Drawing for the job (mm, zero at the part's lowest x, y, z). Give positions to 0.01 mm unless a question says otherwise; leave off trailing zeros. Write each loop counter-clockwise with the first axis right and the second up, starting at its lowest first coordinate (ties: lowest second). Pieces come first, ordered by that corner, then holes.
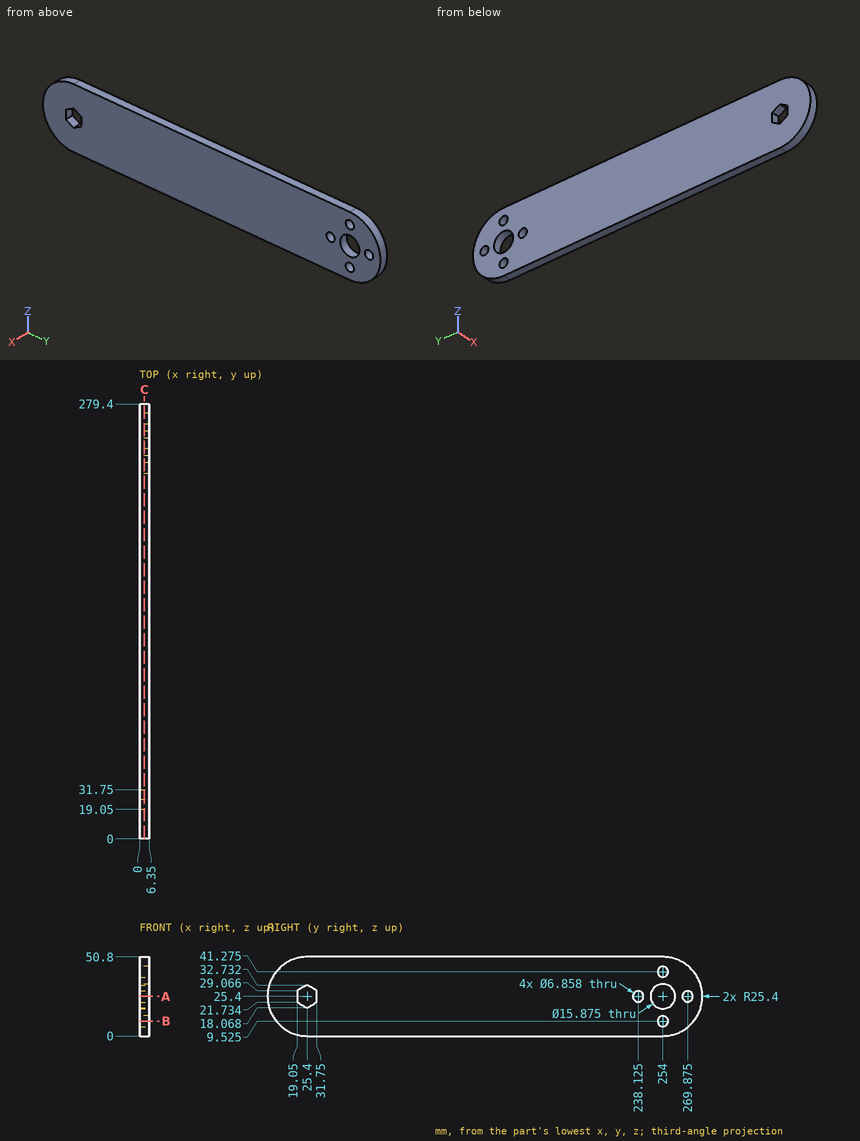
1. Probe probe 1 along Y at (x, z) = (2, 25.4); probe 2 along Y at (x, z) = (5.25, 30) (1 decimal); probe 3 along Y at (x, z) = (5, 41.5) (1 decimal). List the from-to ranges inside material, lowest first.
Calculated:
probe 1: y = 0 to 19.05, 31.75 to 234.7, 241.55 to 246.06, 261.94 to 266.45, 273.3 to 279.4
probe 2: y = 0.4 to 20.7, 30.1 to 247.5, 260.5 to 279
probe 3: y = 5.8 to 250.6, 257.4 to 273.6
2. Slice it at B-B, the plane z = 9.5. Write the cut outline in (x, y).
Calculated:
outline: (0, 5.59) - (6.35, 5.59) - (6.35, 250.57) - (0, 250.57) - close; (0, 257.43) - (6.35, 257.43) - (6.35, 273.81) - (0, 273.81) - close
3. Slice it at C-C, the plane x = 3. State how many separate pieces and enclosed holes the cut face has, and give its area (3 significant figures).
Calculated:
separate pieces: 1
enclosed holes: 6
area: 13,200 mm2
4. Pin check, flat tips, straight feed: P1, Ø3, axis at x = 2.5, z = 5.5, coming from the -Y side; P2, Ø4, axis at y = 269.875, z = 25.4, coming from the -X side; P3, Ø1.9, axis at x = 4.5, z = 27, coming from the -Y side. Stop position of each tip, or through.
Calculated:
P1: stops at y = 7.89
P2: passes through
P3: stops at y = 0.01
5. Slice it at A-A, the plane z = 25.4. Write the cut outline in (x, y).
Calculated:
outline: (0, 0) - (6.35, 0) - (6.35, 19.05) - (0, 19.05) - close; (0, 31.75) - (6.35, 31.75) - (6.35, 234.7) - (0, 234.7) - close; (0, 241.55) - (6.35, 241.55) - (6.35, 246.06) - (0, 246.06) - close; (0, 261.94) - (6.35, 261.94) - (6.35, 266.45) - (0, 266.45) - close; (0, 273.3) - (6.35, 273.3) - (6.35, 279.4) - (0, 279.4) - close
